Autodesk Inventor part; units mm, degrees
ref_plane "YZ Plane" through (0, 0, 0) normal (1, 0, 0) x (0, 1, 0)
ref_plane "XZ Plane" through (0, 0, 0) normal (0, 1, 0) x (-1, 0, 0)
ref_plane "XY Plane" through (0, 0, 0) normal (0, 0, 1) x (1, 0, 0)
sketch "Sketch1" plane through (0, 0, 0) normal (0, 0, 1) x (1, 0, 0)
  line L0 (83, 0) -> (83, 180)
  line L1 (83, 180) -> (0, 180)
  line L2 (0, 180) -> (0, 0)
  line L3 (0, 0) -> (83, 0)
  line L4 (10, 171.8151) -> (10, 9.9445)
  line L5 (73, 174.9264) -> (73, 13.0559)
  circle A0 centre (10, 160) radius 2.1
  circle A1 centre (73, 160) radius 2.1
  circle A2 centre (10, 20) radius 2.1
  circle A3 centre (73, 20) radius 2.1
  dimension "d0" = 83
  dimension "d1" = 180
  dimension "d8" = 4.2
  dimension "d9" = 4.2
  dimension "d10" = 4.2
  dimension "d11" = 4.2
  dimension "d12" = 10
  dimension "d13" = 10
  dimension "d14" = 20
  dimension "d15" = 20
  dimension "d16" = 20
  dimension "d17" = 20
extrude "Extrusion1" add sketch "Sketch1" along normal blind 3
equation "\"d9\" = d8"
equation "\"d10\" = d8"
equation "\"d11\" = d10"
properties part number "BaseC_2" material "PMMA Plastic"
Design review of the part built by this model. Coordinates are the model's own, in mm. Give positions to 0.01 mm unless a question says otherwise; leave off trailing zeros. Loops run counter-clockwise (first coordinate to the right, second up) from the corner with the lowest first, then second, coordinate; pieces in that order, holes last. Notation, with made-up numbers: M 4,83 L 15,83 A34 ccw 15,117 Z; hole C -17.75,57.25 d6. An arc over 180 degrees is marked long. Return JSON: item names as keys, results as strings. Group by question number.
Item 1: We need section B-B (x = 10). Give the boundary of the cut face in (y, z).
Item 2: We need section A-A (y = 20). Give the boundary of the cut face in (x, z).
Item 3: For probe 1 along X at (y, z) = (160, 1.45); probe 2 along Y at (x, z) = (10, 0.8); probe 3 along X at (y, z) = (19.5, 2.15), list the stretches that pass through material, from the lowest coordinate up.
Item 4: Mouldability with a two-part tool opening along Y and no side actions: class faces 1 (the flat face through (41, 0, 1)), 2 (the cylindrical face through (72.727, 157.918, 1.479)), 3 (the flat face through (41, 91, 3)) as released by +Y, released by -Y, zero draft, split by the parting line, or undercut.
Output:
{
 "1": {"outline": "M 0,0 L 17.9,0 L 17.9,3 L 0,3 Z; M 22.1,0 L 157.9,0 L 157.9,3 L 22.1,3 Z; M 162.1,0 L 180,0 L 180,3 L 162.1,3 Z"},
 "2": {"outline": "M 0,0 L 7.9,0 L 7.9,3 L 0,3 Z; M 12.1,0 L 70.9,0 L 70.9,3 L 12.1,3 Z; M 75.1,0 L 83,0 L 83,3 L 75.1,3 Z"},
 "3": {"probe 1": "x = 0 to 7.9, 12.1 to 70.9, 75.1 to 83", "probe 2": "y = 0 to 17.9, 22.1 to 157.9, 162.1 to 180", "probe 3": "x = 0 to 7.96, 12.04 to 70.96, 75.04 to 83"},
 "4": {"face 1": "released by -Y", "face 2": "undercut", "face 3": "zero draft"}
}
